The listing builds one solid part. Answer for the finished solid, in the listing's coordinates (mm). A direction names the side the tool comes from. Round coordinates to 2 decimals unless told otherwise and drop trailing zeros. Loops run counter-clockwise (first coordinate to the right, second up) from the corner with the lowest first, then second, coordinate; pieces in that order, holes last. Notation, with made-up numbers: M 37,-36 L 58,-36 A5 cw 58,-27 Z; hole C 64,-30 d1. An arc over 180 degrees is marked long. Answer as a JSON object with one key per item and string values.
```python
from build123d import *

# Parameters (mm, degrees)
CROQUIS1_W              = 10
CROQUIS1_H              = 20
CROQUIS1_R              = 1.6
SALIENTE_EXTRUIR1_DEPTH = 5
CORTAR_EXTRUIR1_DEPTH   = 3
REDONDEO1_R             = 2


with BuildPart() as part:
    # Croquis1 → Saliente-Extruir1 (new body)
    with BuildSketch(Plane(origin=(0, 0, 0), x_dir=(1, 0, 0), z_dir=(0, 1, 0))):
        Rectangle(CROQUIS1_W, CROQUIS1_H)
        with Locations((0, 4.474482181)):
            Circle(CROQUIS1_R, mode=Mode.SUBTRACT)
        with Locations((0, -4.474482181)):
            Circle(CROQUIS1_R, mode=Mode.SUBTRACT)
    extrude(amount=SALIENTE_EXTRUIR1_DEPTH)

    # Croquis2 → Cortar-Extruir1 (cut)
    with BuildSketch(Plane.XZ):
        Polygon((3.233161507, 4.474482181), (1.616580754, 7.274482181), (-1.616580754, 7.274482181), (-3.233161507, 4.474482181), (-1.616580754, 1.674482181), (1.616580754, 1.674482181), align=None)
        Polygon((1.616580754, -1.674482181), (3.233161507, -4.474482181), (1.616580754, -7.274482181), (-1.616580754, -7.274482181), (-3.233161507, -4.474482181), (-1.616580754, -1.674482181), align=None)
    extrude(amount=-CORTAR_EXTRUIR1_DEPTH, mode=Mode.SUBTRACT)

    # Redondeo1
    redondeo1_edges = [part.edges().sort_by_distance(p)[0] for p in [
        (5, 2.5, 10),
        (-5, 2.5, 10),
        (-5, 2.5, -10),
        (5, 2.5, -10),
    ]]
    fillet(redondeo1_edges, radius=REDONDEO1_R)


solid = part.part
```
Item 1: The part is cut by section D-D (y = 1.6). Give the vertices of the cut face in (x, z).
Values follow:
{"outline": "M -5,-8 A2 ccw -3,-10 L 3,-10 A2 ccw 5,-8 L 5,8 A2 ccw 3,10 L -3,10 A2 ccw -5,8 Z; hole M -3.23,-4.47 L -1.62,-7.27 L 1.62,-7.27 L 3.23,-4.47 L 1.62,-1.67 L -1.62,-1.67 Z; hole M -3.23,4.47 L -1.62,1.67 L 1.62,1.67 L 3.23,4.47 L 1.62,7.27 L -1.62,7.27 Z"}
Item 2: A flat-ended cylindrical pin translates along its axis: P1, Ø5, axis at x = 0, z = -4.47, coming from the -Y side. Find the tip coordinate at first contact, or state that the pin passes through.
Values follow:
{"P1": "y = 3"}
Item 3: The part is cut by section A-A (y = 3.6). Give the vertices of the cut face in (x, z), then the cut area to 3 significant figures.
Values follow:
{"outline": "M -5,-8 A2 ccw -3,-10 L 3,-10 A2 ccw 5,-8 L 5,8 A2 ccw 3,10 L -3,10 A2 ccw -5,8 Z; hole C 0,-4.47 d3.2; hole C 0,4.47 d3.2", "area": "180 mm^2"}
Item 4: Which of the six approach directions +Z, -Z, +X, -X, +Y, -Y give full straight-line access (tool end or side, diameter ignored) to faces 1 (the face through (4.4, 2.54, 9.43)), 2 (the face through (0, 1, -1.674))?
Values follow:
{"face 1": "+Z, +X, +Y, -Y", "face 2": "-Y"}
Item 5: Straight lines are drawn through the part: line 1 (Z direction, x = 0, y = 4.45); line 2 (Z direction, x = 0.5, y = 2.6); line 3 (Y direction, x = -2, z = -6). For each, find the intervals that lie inside material, in ascending order.
Values follow:
{"line 1": "-10 to -6.07, -2.87 to 2.87, 6.07 to 10", "line 2": "-10 to -7.27, -1.67 to 1.67, 7.27 to 10", "line 3": "3 to 5"}
Item 6: The part is cut by section C-C (z = 5.75). Give the vertices of the cut face in (x, y), then the cut area to 3 significant figures.
Values follow:
{"outline": "M -5,0 L -2.5,0 L -2.5,3 L -0.97,3 L -0.97,5 L -5,5 Z; M 0.97,3 L 2.5,3 L 2.5,0 L 5,0 L 5,5 L 0.97,5 Z", "area": "31.2 mm^2"}
Item 7: Determine the mould class of faces 3 (the face through (0, 2, 10)), 4 (the face through (-4.43, 2.54, -9.4)), 5 (the face through (0, 0, 0)), 6 (the face through (-2.436, 1.479, 3.094)) for opening direction Z: released by +Z, released by -Z, zero draft, split by the parting line, or undercut.
Values follow:
{"face 3": "released by +Z", "face 4": "released by -Z", "face 5": "zero draft", "face 6": "undercut"}
Item 8: The part is cut by section B-B (x = 0). Give the vertices of the cut face in (y, z).
Values follow:
{"outline": "M 0,-10 L 5,-10 L 5,-6.07 L 3,-6.07 L 3,-7.27 L 0,-7.27 Z; M 0,-1.67 L 3,-1.67 L 3,-2.87 L 5,-2.87 L 5,2.87 L 3,2.87 L 3,1.67 L 0,1.67 Z; M 0,7.27 L 3,7.27 L 3,6.07 L 5,6.07 L 5,10 L 0,10 Z"}
